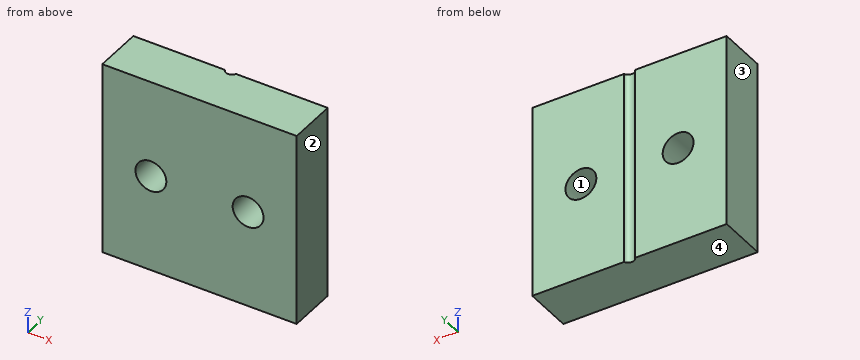
```python
from build123d import *

# Parameters (mm, degrees)
SKETCH1_W           = 20
SKETCH1_H           = 20
BOSS_EXTRUDE1_DEPTH = 5
SKETCH2_R           = 0.6223
CUT_EXTRUDE1_DEPTH  = 65.157116795
SKETCH3_R           = 1.5875
CUT_EXTRUDE2_DEPTH  = 81.174749068


with BuildPart() as part:
    # Sketch1 → Boss-Extrude1 (new body)
    with BuildSketch(Plane(origin=(0, 0, 0), x_dir=(1, 0, 0), z_dir=(0, 1, 0))):
        with Locations((-50.754716981, 42.075471698)):
            Rectangle(SKETCH1_W, SKETCH1_H)
    extrude(amount=BOSS_EXTRUDE1_DEPTH)

    # Sketch2 → Cut-Extrude1 (cut, through all)
    with BuildSketch(Plane.XY.offset(-32.075471698)):
        with Locations((-50.754716981, 5.25)):
            Circle(SKETCH2_R)
    extrude(amount=-CUT_EXTRUDE1_DEPTH, mode=Mode.SUBTRACT)

    # Sketch3 → Cut-Extrude2 (cut, through all)
    with BuildSketch(Plane(origin=(0, 5, 0), x_dir=(1, 0, 0), z_dir=(0, 1, 0))):
        with Locations(Location((-55.754716981, 42.075471698, 0), (0, 0, 270))):
            Circle(SKETCH3_R)
        with Locations(Location((-45.754716981, 42.075471698, 0), (0, 0, 270))):
            Circle(SKETCH3_R)
    extrude(amount=-CUT_EXTRUDE2_DEPTH, mode=Mode.SUBTRACT)


solid = part.part
```
The listing builds one solid part. Answer for the finished solid, in the listing's coordinates (mm). Face numbers are marked on the shaded views. Coordinates: 2 decimals unless noted, no trailing zeros. Write each loop counter-clockwise with the first axis right and the second up, starting at its lowest first coordinate (ties: lowest second). Pieces come first, ordered by that corner, then holes. Notation, with made-up numbers: M -1,61 L 51,61 A28 ccw 51,90 Z; hole C 76.5,-24 d11. An arc over 180 degrees is marked long. Use a Markdown table: item, result. Add a question column.
1. Section B-B (x = -50.5) is taken. Give the vertices of the cut face in (y, z).
2. Straight lines are drawn through the part: line 1 along Z through (x, y) = (-44.5, 0.7); line 2 along Z through (x, y) = (-55, 0.6). For each, find the intervals that lie inside material, in ascending order. Write a range as [from, to].
3. Section A-A (y = 1) is taken. Give the vertices of the cut face in (x, z) (1 decimal), plus the area to 3 significant figures.
4. For a pull along X with two mould halves and no side action, classify the marked faces 1, 2, 3 and 4 as +X half, -X half, draft (parallel to the pull), parting line (faces both ways), or undercut.
Data:
| question | item | result |
|---|---|---|
| 1 | outline | M 0,-52.08 L 4.68,-52.08 L 4.68,-32.08 L 0,-32.08 Z |
| 2 | line 1 | z = [-52.08, -43.05], [-41.1, -32.08] |
| 2 | line 2 | z = [-52.08, -43.47], [-40.68, -32.08] |
| 3 | outline | M -60.8,-52.1 L -40.8,-52.1 L -40.8,-32.1 L -60.8,-32.1 Z; hole C -55.8,-42.1 d3.2; hole C -45.8,-42.1 d3.2 |
| 3 | area | 384 mm2 |
| 4 | face 1 | undercut |
| 4 | face 2 | +X half |
| 4 | face 3 | -X half |
| 4 | face 4 | draft |
